from build123d import *

# Parameters (mm, degrees)
CROQUIS1_R                   = 75
SALIENTE_EXTRUIR1_DEPTH      = 10
CROQUIS2_R                   = 37.5
CROQUIS4_R                   = 37.5
SALIENTE_EXTRUIR3_DEPTH      = 381
SALIENTE_EXTRUIR4_DEPTH      = 100
SALIENTE_EXTRUIR4_DEPTH_BACK = 100
CROQUIS6_W                   = 141.368041576
CROQUIS6_H                   = 480.917106318
CORTAR_EXTRUIR1_DEPTH        = 20


with BuildPart() as part:
    # Croquis1 → Saliente-Extruir1 (new body)
    with BuildSketch(Plane.XY):
        Circle(CROQUIS1_R)
    extrude(amount=SALIENTE_EXTRUIR1_DEPTH)

    # Barrer2: sweep along a curve in space
    with BuildLine() as barrer2_path:
        Line((0, 0, 0), (0, 192.014551033, 534.190633363))
        ThreePointArc((0, 192.014551033, 534.190633363), (0, 211.131156127, 630.926630457), (0, 200.813232001, 728.992109428))
        Line((0, 200.813232001, 728.992109428), (0, 0, 1500))
    # Croquis2 → Barrer2 (sweep)
    with BuildSketch(Plane.XY.offset(10)):
        Circle(CROQUIS2_R)
    sweep(path=barrer2_path.line)

    # Croquis4 → Saliente-Extruir3 (add)
    with BuildSketch(Plane(origin=(0, 0, 0), x_dir=(-1, 0, 0), z_dir=(0, 0, -1))):
        with Locations(Location((0, 0, 0), (0, 0, 180))):
            Circle(CROQUIS4_R)
    extrude(amount=SALIENTE_EXTRUIR3_DEPTH)

    # Croquis5 → Saliente-Extruir4 (add, two sides: drawn at the far end of the back side and taken through both)
    with BuildSketch(Plane(origin=(0, 0, 0), x_dir=(0, 0, -1), z_dir=(1, 0, 0)).offset(-SALIENTE_EXTRUIR4_DEPTH_BACK)):
        with BuildLine():
            Line((-1476.800956395, -33.919933481), (-1476.800956395, 39.013652266))
            Line((-1476.800956395, 39.013652266), (-1525.449183366, 87.661879237))
            ThreePointArc((-1525.449183366, 87.661879237), (-1561.135751737, 111.506881882), (-1603.230929297, 119.880133306))
            Line((-1603.230929297, 119.880133306), (-1792.167323705, 119.880133306))
            ThreePointArc((-1792.167323705, 119.880133306), (-1863.764639403, 112.019581969), (-1931.951080097, 88.812402305))
            Line((-1931.951080097, 88.812402305), (-1975.041969043, 68.662666235))
            ThreePointArc((-1975.041969043, 68.662666235), (-2021.25202894, 28.071923633), (-2038.447383579, -30.981423431))
            Line((-2038.447383579, -30.981423431), (-2038.447383579, -33.919933481))
            Line((-2038.447383579, -33.919933481), (-1476.800956395, -33.919933481))
        make_face()
    extrude(amount=SALIENTE_EXTRUIR4_DEPTH + SALIENTE_EXTRUIR4_DEPTH_BACK)

    # Croquis6 → Cortar-Extruir1 (cut)
    with BuildSketch(Plane.XZ.offset(33.919933481)):
        with Locations((0, 1764.64048311)):
            Rectangle(CROQUIS6_W, CROQUIS6_H)
    extrude(amount=-CORTAR_EXTRUIR1_DEPTH, mode=Mode.SUBTRACT)


solid = part.part
The model under review builds one solid part; all positions refer to its coordinate system, in mm. A direction names the side the tool comes from. Give positions to 0.01 mm unless a question says otherwise; leave off trailing zeros. Write each loop counter-clockwise with the first axis right and the second up, starting at its lowest first coordinate (ties: lowest second). Pieces come first, ordered by that corner, then holes. Notation, with made-up numbers: M -3,83.5 L 44,83.5 A21 ccw 44,120.5 Z; hole C -28,-2 d10. An arc over 180 degrees is marked long. One line per question, with ' | ' between items. Start each with the question number.
Item 1: Wall thickness on line 1 (Z direction, x = 58.5, y = -24.5); line 2 (Z direction, x = -45, y = 46.5); line 3 (Z direction, x = 66, y = 13.5): over which ranges is each line inside the solid? List them lowest first. Write a range as from..to.
Item 2: For pin 1 (22 mm diameter, centred on x = -59.5, y = 18, fed in from -Z); pin 2 (12 mm diameter, centred on y = 91.5, z = 1212, fed in from -X); pin 3 (3 mm diameter, centred on x = -21.5, y = 70.5, fed in from +Z), all flat-tipped, find the tip position at first contact; note any pin that passes through.
Item 3: We need section A-A on z = 1892.5. Write out the cut boundary in (x, y).
Item 4: For faces 1 (the cylindrical face through (-1.4, 111.274, 1560.578)), 2 (the cylindrical face through (17.3, 33.27, -187.83)), 3 (the flat face through (15.6, 34.4, 10)), list the 3-axis set-ups (+Z, -Z, +X, -X, +Y, -Y) from which the entire face can be reached by the end or side of a thin tool; tool diameter is ignored.
Item 5: Draft analysis for pull direction X (two halves, no side actions). For faces 4 (the flat face through (-1.4, 78.88, 1953.19)), 5 (the flat face through (-100, 44, 1762)), 6 (the flat face through (-1, -13.92, 1768)), state which applies: released by +X, released by -X, zero draft, split by the parting line, or undercut.
Results found:
1) line 1: z = 0..10, 1476.8..1524.18, 2005.1..2038.26 | line 2: z = 0..10, 1484.29..2006.53 | line 3: z = 0..10, 1476.8..2029.05
2) pin 1: stops at z = 0 | pin 2: stops at x = -34.72 | pin 3: stops at z = 1974.32
3) outline: M -100,-33.92 L -70.68,-33.92 L -70.68,-13.92 L 70.68,-13.92 L 70.68,-33.92 L 100,-33.92 L 100,104.26 L -100,104.26 Z
4) face 1: +X, -X, +Y | face 2: -Z | face 3: none
5) face 4: zero draft | face 5: released by -X | face 6: undercut
